The listing builds one solid part. Answer for the finished solid, in the listing's coordinates (mm). A direction names the side the tool comes from. Coordinates: 2 decimals unless noted, no trailing zeros. Loops run counter-clockwise (first coordinate to the right, second up) from the corner with the lowest first, then second, coordinate; pieces in that order, holes last. Notation, with made-up numbers: M 77.5,21 L 133.5,21 A27 ccw 133.5,41 Z; hole C -9.75,-19 d10. An arc over 180 degrees is marked long. Answer as a JSON object with one key per item and string values. Group by question number.
1. Given pin 1 (12 mm diameter, centred on x = 12.5, z = 15.5, fed in from +Y); pin 2 (3.5 mm diameter, centred on y = 17, z = -4, fed in from -X); pin 3 (3.5 mm diameter, centred on y = 17, z = 2.5, fed in from +X); pin 4 (4 mm diameter, centred on x = 3.5, y = 17, fed in from -Z), each flat-ended and moving along its own axis, determine where each tip first touches the part or whether it passes through.
2. A cutting plane is placed at C-C on z = -2. Give the vertices of the cut face in (x, y), and give its area (3 significant figures).
3. A cutting plane is placed at B-B on y = 10. Give the vertices of the cut face in (x, z).
4. A cutting plane is placed at D-D on x = 8.5. Give the vertices of the cut face in (y, z), and give its area (3 significant figures).
5. For faces 4 (the face through (-20, 7.5, -9.4)), 5 (the face through (-14.993, 17, -1)), 6 (the face through (23.881, 8, 9)), 7 (the face through (14, 17, -2)), determine the directions among +Z, -Z, +X, -X, +Y, -Y from which every point of the face is accessible in a straight line to the end or side of a thin tool.
6. Determine the mould class of faces 1 (the face through (24.1, 7.6, -3)), 2 (the face through (0, 0, 5)), 3 (the face through (0, 8, -9)) for opening direction Y: released by +Y, released by -Y, zero draft, split by the parting line, or undercut.
7. Straight lines are drawn through the part: L1, parallel to Y at x = -2, z = -3.75; L2, parallel to Y at x = 13.5, z = 8.5; L3, parallel to X at y = 9.5, z = -1. For each, find the intervals that lie inside material, in ascending order.
8. A cutting plane is placed at A-A on z = -6. Give the vertices of the cut face in (x, y), and give its area (3 significant figures).
Autodesk Fusion 360 part; units mm, degrees
sketch "スケッチ1" plane through (0, 0, 0) normal (0, 1, 0) x (1, 0, 0)
  line L0 (-25, 10) -> (25, 10)
  line L1 (25, 10) -> (25, -20)
  line L2 (25, -20) -> (-25, -20)
  line L3 (-25, -20) -> (-25, 10)
  dimension "d1" = 50
extrude "押し出し1" add sketch "スケッチ1" along normal blind 15
sketch "スケッチ2" plane through (0, 0, 20) normal (0, 0, 1) x (1, 0, 0)
  line L0 (-25, 0) -> (25, 0)
  line L1 (25, 0) -> (25, 15)
  line L2 (25, 15) -> (-25, 15)
  line L3 (-25, 15) -> (-25, 0)
  line L4 (-24.1188, 14.0157) -> (23.8812, 14.0157)
  line L5 (23.8812, 14.0157) -> (23.8812, 1.0157)
  line L6 (23.8812, 1.0157) -> (-24.1188, 1.0157)
  line L7 (-24.1188, 1.0157) -> (-24.1188, 14.0157)
  dimension "d4" = 48
  dimension "d5" = 13
extrude "押し出し2" cut sketch "スケッチ2" against normal blind 29 contours L4 L5 L6 L7
sketch "スケッチ3" plane through (0, 15, 0) normal (0, 1, 0) x (-1, 0, 0)
  line L0 (25, 20) -> (-25, 20)
  line L1 (-25, 20) -> (-25, -10)
  line L2 (-25, -10) -> (25, -10)
  line L3 (25, -10) -> (25, 20)
  line L4 (25, -10) -> (20, -10)
  line L5 (20, -10) -> (20, -3)
  line L6 (20, -3) -> (25, -3)
  line L7 (25, -3) -> (25, -10)
  dimension "d8" = 5
  dimension "d9" = 7
extrude "押し出し3" cut sketch "スケッチ3" against normal blind 25 contours L2 L3 L4 L5 L6 L7
sketch "スケッチ4" plane through (0, 15, 0) normal (0, 1, 0) x (-1, 0, 0)
  line L0 (20, -10) -> (20, -3)
  line L1 (20, -3) -> (25, -3)
  line L2 (25, -3) -> (25, 20)
  line L3 (25, 20) -> (-25, 20)
  line L4 (-25, 20) -> (-25, -10)
  line L5 (-25, -10) -> (20, -10)
  line L6 (-25, -10) -> (-20, -10)
  line L7 (-20, -10) -> (-20, -3)
  line L8 (-20, -3) -> (-25, -3)
  line L9 (-25, -3) -> (-25, -10)
  dimension "d12" = 7
  dimension "d13" = 5
extrude "押し出し4" cut sketch "スケッチ4" against normal blind 65 contours L4 L5 L6 L7 L8 L9
sketch "スケッチ5" plane through (0, 15, 0) normal (0, 1, 0) x (-1, 0, 0)
  line L0 (-25, -3) -> (-20, -3)
  line L1 (-20, -3) -> (-20, -10)
  line L2 (-20, -10) -> (20, -10)
  line L3 (20, -10) -> (20, -3)
  line L4 (20, -3) -> (25, -3)
  line L5 (25, -3) -> (25, 20)
  line L6 (25, 20) -> (-25, 20)
  line L7 (-25, 20) -> (-25, -3)
  line L8 (14.9932, -10) -> (-15.0068, -10)
  line L9 (-15.0068, -10) -> (-15.0068, 8)
  line L10 (-15.0068, 8) -> (14.9932, 8)
  line L11 (14.9932, 8) -> (14.9932, -10)
  dimension "d16" = 30
  dimension "d17" = 18
extrude "押し出し5" add sketch "スケッチ5" along normal blind 4 contours L2 L8 L9 L10 L11
sketch "スケッチ6" plane through (0, 0, -10) normal (0, 0, -1) x (-1, 0, 0)
  line L0 (-20, 15) -> (-20, 0)
  line L1 (-20, 0) -> (20, 0)
  line L2 (20, 0) -> (20, 15)
  line L3 (20, 15) -> (14.9932, 15)
  line L4 (14.9932, 15) -> (14.9932, 19)
  line L5 (14.9932, 19) -> (-15.0068, 19)
  line L6 (-15.0068, 19) -> (-15.0068, 15)
  line L7 (-15.0068, 15) -> (-20, 15)
  line L8 (14, 18) -> (-14, 18)
  line L9 (-14, 18) -> (-14, 15)
  line L10 (-14, 15) -> (14, 15)
  line L11 (14, 15) -> (14, 18)
  line L12 (-15.0068, 15) -> (14.9932, 15)
  line L13 (25, 15) -> (-25, 15)
extrude "押し出し6" cut sketch "スケッチ6" against normal blind 17 contours L8 L9 L10 L11 L12 L13
From the geometry:
{
 "1": {"pin 1": "stops at y = 15", "pin 2": "stops at x = -14.99", "pin 3": "stops at x = 15.01", "pin 4": "stops at z = -10"},
 "2": {"outline": "M -25,0 L 25,0 L 25,15 L 15.01,15 L 15.01,19 L -14.99,19 L -14.99,15 L -25,15 Z; hole M -24.12,1.02 L 23.88,1.02 L 23.88,14.02 L -24.12,14.02 Z; hole M -14,15 L 14,15 L 14,18 L -14,18 Z", "area": "162 mm²"},
 "3": {"outline": "M -25,-3 L -24.12,-3 L -24.12,20 L -25,20 Z; M -20,-10 L 20,-10 L 20,-9 L -20,-9 Z; M 23.88,-3 L 25,-3 L 25,20 L 23.88,20 Z"},
 "4": {"outline": "M 0,-10 L 15,-10 L 15,7 L 18,7 L 18,-10 L 19,-10 L 19,8 L 15,8 L 15,20 L 14.02,20 L 14.02,-9 L 1.02,-9 L 1.02,20 L 0,20 Z", "area": "94.0 mm²"},
 "5": {"face 4": "-Z, -X, +Y, -Y", "face 5": "+Z, -Z, -X, +Y", "face 6": "+Z, -Z", "face 7": "-Z"},
 "6": {"face 1": "zero draft", "face 2": "released by -Y", "face 3": "undercut"},
 "7": {"L1": "y = 0 to 1.02, 14.02 to 15, 18 to 19", "L2": "y = 0 to 1.02, 14.02 to 15", "L3": "x = -25 to -24.12, 23.88 to 25"},
 "8": {"outline": "M -20,0 L 20,0 L 20,1.02 L -20,1.02 Z; M -20,14.02 L 20,14.02 L 20,15 L 15.01,15 L 15.01,19 L -14.99,19 L -14.99,15 L -20,15 Z; hole M -14,15 L 14,15 L 14,18 L -14,18 Z", "area": "116 mm²"}
}
